from build123d import *

# Parameters (mm, degrees)
SKETCH1_W           = 30
SKETCH1_H           = 15
BOSS_EXTRUDE1_DEPTH = 2
FILLET1_R           = 5
CUT_EXTRUDE1_DEPTH  = 1


with BuildPart() as part:
    # Sketch1 → Boss-Extrude1 (new body)
    with BuildSketch(Plane(origin=(0, 0, 0), x_dir=(1, 0, 0), z_dir=(0, 1, 0))):
        Rectangle(SKETCH1_W, SKETCH1_H)
    extrude(amount=BOSS_EXTRUDE1_DEPTH)

    # Fillet1
    fillet1_edges = [part.edges().sort_by_distance(p)[0] for p in [
        (-15, 1, -7.5),
        (15, 1, -7.5),
        (15, 1, 7.5),
        (-15, 1, 7.5),
    ]]
    fillet(fillet1_edges, radius=FILLET1_R)

    # Sketch3 → Cut-Extrude1 (cut)
    # profile 1 of 2: a face of its own
    with BuildSketch(Plane(origin=(0, 2, 0), x_dir=(1, 0, 0), z_dir=(0, 1, 0))):
        Polygon((-11.70625, 3.379166667), (-10.471527778, 3.379166667), (-10.471527778, -2.265277778), (-8.53125, -2.265277778), (-8.53125, -3.5), (-11.70625, -3.5), align=None)
    # profile 2 of 2: a face of its own
    with BuildSketch(Plane(origin=(0, 2, 0), x_dir=(1, 0, 0), z_dir=(0, 1, 0))):
        with BuildLine():
            Line((7.7375, 3.379166667), (9.176171875, 3.379166667))
            add(Edge.make_bspline(
                [(9.176171875, 3.379166667), (9.271267648, 3.378829131), (9.454163607, 3.378179956), (9.717889589, 3.367937683), (9.960158173, 3.35368472), (10.181328057, 3.33193432), (10.381304623, 3.303095918), (10.560288293, 3.269100215), (10.718273835, 3.230354823), (10.856593641, 3.182075007), (10.981420425, 3.127616107), (11.097776343, 3.065041832), (11.208228378, 2.995048967), (11.312038278, 2.91579581), (11.410108175, 2.828708105), (11.502623084, 2.733698191), (11.588275684, 2.629960422), (11.666535611, 2.51815029), (11.737863234, 2.400528594), (11.800901893, 2.276933841), (11.852165035, 2.147280077), (11.897461517, 2.01344108), (11.930087105, 1.873503596), (11.952777724, 1.728829939), (11.969390908, 1.578910842), (11.970346086, 1.477062464), (11.970833333, 1.425108507)],
                knots=[0, 0, 0, 0, 1.749336639, 3.364467119, 4.854658419, 6.213483162, 7.451590619, 8.570285859, 9.5643256, 10.440900261, 11.26203566, 12.067320669, 12.869050712, 13.665104639, 14.467235401, 15.27997916, 16.102287765, 16.939272006, 17.78853747, 18.631303466, 19.488103222, 20.351255419, 21.228522269, 22.127379805, 23.044756219, 24, 24, 24, 24], degree=3))
            add(Edge.make_bspline(
                [(11.970833333, 1.425108507), (11.969567641, 1.370880511), (11.967085849, 1.264549293), (11.953717567, 1.108357407), (11.929284548, 0.958923936), (11.892277185, 0.816686402), (11.849742029, 0.679874494), (11.793181181, 0.551012476), (11.729346675, 0.428226238), (11.653532296, 0.313252637), (11.57032972, 0.203537881), (11.473566874, 0.103285547), (11.369512504, 0.007107453), (11.252317335, -0.078972131), (11.12714744, -0.160773597), (10.991515824, -0.234907509), (10.846307665, -0.303237424), (10.744219138, -0.341342904), (10.692013889, -0.360828993)],
                knots=[0, 0, 0, 0, 1.099860209, 2.156625411, 3.176576793, 4.16617041, 5.135385252, 6.078461593, 7.016046972, 7.938469504, 8.868247731, 9.803980173, 10.76021508, 11.73834243, 12.748633912, 13.790971185, 14.870363756, 16, 16, 16, 16], degree=3))
            Line((10.692013889, -0.360828993), (12.279513889, -3.5))
            Line((12.279513889, -3.5), (10.906987847, -3.5))
            Line((10.906987847, -3.5), (9.391145833, -0.501388889))
            Line((9.391145833, -0.501388889), (8.972222222, -0.501388889))
            Line((8.972222222, -0.501388889), (8.972222222, -3.5))
            Line((8.972222222, -3.5), (7.7375, -3.5))
            Line((7.7375, -3.5), (7.7375, 3.379166667))
        make_face()
        with BuildLine():
            Line((8.972222222, 0.733333333), (9.453157552, 0.733333333))
            add(Edge.make_bspline(
                [(9.453157552, 0.733333333), (9.511955894, 0.73399556), (9.624542084, 0.735263581), (9.786455813, 0.74114519), (9.933512094, 0.75531696), (10.066342435, 0.773222462), (10.185615227, 0.793896951), (10.290266598, 0.823524747), (10.381909067, 0.855271682), (10.459456666, 0.894724886), (10.525711554, 0.939591736), (10.582918408, 0.990561593), (10.630236679, 1.049552713), (10.66918203, 1.11496197), (10.699477279, 1.187367895), (10.721590489, 1.265975634), (10.733948504, 1.35168063), (10.735370336, 1.410828747), (10.736111111, 1.441644965)],
                knots=[0, 0, 0, 0, 1.688639943, 3.233382647, 4.650958383, 5.928841754, 7.082724185, 8.122798841, 9.049171256, 9.863274652, 10.613301712, 11.341792392, 12.054588806, 12.776240173, 13.521029143, 14.301969904, 15.115324896, 16, 16, 16, 16], degree=3))
            add(Edge.make_bspline(
                [(10.736111111, 1.441644965), (10.734710607, 1.478102802), (10.731959577, 1.549717465), (10.704660808, 1.652817469), (10.661207064, 1.748243577), (10.601643884, 1.835564629), (10.526631801, 1.912116292), (10.440549519, 1.979597192), (10.341539172, 2.032956039), (10.249863042, 2.068150966), (10.166459192, 2.089208454), (10.091189849, 2.104900308), (10.004027496, 2.116021575), (9.904906331, 2.127817658), (9.794079017, 2.135466821), (9.670941479, 2.141049186), (9.535847367, 2.143333205), (9.44167394, 2.144063366), (9.392523872, 2.144444444)],
                knots=[0, 0, 0, 0, 1.020303359, 2.004196876, 2.966617323, 3.9489082, 4.950758222, 5.960522915, 7.003732012, 8.091992268, 8.70421221, 9.413913587, 10.24622431, 11.166358409, 12.212345909, 13.359657661, 14.621978493, 16, 16, 16, 16], degree=3))
            Line((9.392523872, 2.144444444), (8.972222222, 2.144444444))
            Line((8.972222222, 2.144444444), (8.972222222, 0.733333333))
        make_face(mode=Mode.SUBTRACT)
    extrude(amount=-CUT_EXTRUDE1_DEPTH, mode=Mode.SUBTRACT)


solid = part.part
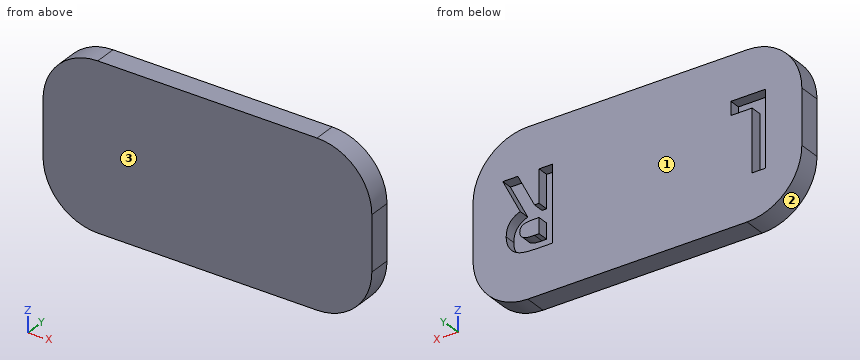
The listing builds one solid part. Answer for the finished solid, in the listing's coordinates (mm). Face numbers are marked on the shaded views. Round coordinates to 2 decimals unless told otherwise and drop trailing zeros. Write each loop counter-clockwise with the first axis right and the second up, starting at its lowest first coordinate (ties: lowest second). Pieces come first, ordered by that corner, then holes. Notation, with made-up numbers: M 18.5,36.25 L 41.5,36.25 A21 cw 41.5,55.25 Z; hole C 65.25,48 d1. An arc over 180 degrees is marked long. Write each question's results on one line, items separated by ' | '. Start each with the question number.
(1) The part is cut by section A-A, the plane y = 1.45. Give the number of separate pieces and of enclosed holes in the cut face, and give its area (3 significant figures).
(2) Find the intervals of material crossed by line 1 (X direction, y = 1.15, z = 3); line 2 (X direction, y = 1.3, z = 1.75); line 3 (Z direction, x = 9.5, y = 1.1), in increasing order.
(3) This flat-tipped pin is pushed along its axis until it touches: P1, Ø0.8, axis at x = 11.5, y = 1.5, coming from the -Z side. Where does it stop, or does it pass through?
(4) The part is cut by section C-C, the plane x = -13. Write down the section's boundary in (y, z), and give its area (3 significant figures).
(5) Determine the mould class of the marked faces 1, 2 and 3 for opening direction Y: +Y half, -Y half, draft (parallel to the pull), parting line (faces both ways), or undercut.
(6) The part is cut by section B-B, the plane z = 1.5. Write down the section's boundary in (x, y).
(7) The part is cut by section D-D, the plane z = 6.5. Write down the section's boundary in (x, y), and give its area (3 significant figures).
Worked answers:
1) separate pieces: 2 | enclosed holes: 2 | area: 397 mm²
2) line 1: x = -14.97 to -11.71, -8.53 to 7.74, 8.97 to 10.65, 12.03 to 14.97 | line 2: x = -15 to -11.71, -10.47 to 7.74, 8.97 to 10.02, 11.39 to 15 | line 3: z = -7.5 to -3.38, -2.14 to -0.73, 0.72 to 7.5
3) P1: stops at z = -7.38
4) outline: M 0,-6.5 L 2,-6.5 L 2,6.5 L 0,6.5 Z | area: 26.0 mm²
5) face 1: +Y half | face 2: draft | face 3: -Y half
6) outline: M -15,0 L 15,0 L 15,2 L 11.27,2 L 11.27,1 L 9.9,1 L 9.9,2 L 8.97,2 L 8.97,1 L 7.74,1 L 7.74,2 L -10.47,2 L -10.47,1 L -11.71,1 L -11.71,2 L -15,2 Z
7) outline: M -13,0 L 13,0 L 13,2 L -13,2 Z | area: 52.0 mm²
